Verification items for the finished model (mm, model axes). A direction names the side the tool comes from. Coordinates: 2 decimals unless noted, no trailing zeros. Order: outer loops, then holes, each group sorted by start corner. A loop starts at its lowest first (then second) coordinate and runs counter-clockwise, first axis right, second up. Notation, with made-up numbers: M 88,-20 L 139,-20 A35 cw 139,18 Z; hole C -18.5,-30 d10. An arc over 180 degrees is marked long. Answer as a JSON object with one key per item and string values. Group by question number.
(1) Material ranges on line 1 (X direction, y = 0, z = 1.65); line 2 (Y direction, x = 35, z = 2.35); line 3 (X direction, y = 0.7, z = 4.4), recorded low to high.
(2) Cross-section at A-A (x = 0). Enter the section's corners in (y, z), plus the area to 3 significant figures.
(3) Access from +Z, -Z, +X, -X, +Y, -Y to the whole of each face (thin tool, end or side, straight path). Record for faces 4 (the face through (-42.5, -0.1, 2.5)), 5 (the face through (-1, -1, 3)).
(4) Cross-section at C-C (y = 0). Count the separate pieces of the cut face and the enclosed holes in it, plus the area to 3 significant figures.
(5) Cross-section at B-B (z = 2). Enter the section's corners in (x, y).
(6) Mould release check, pull along Y, two halves, no side actions. Record for faces 1 (the face through (34, -1, 3)), 2 (the face through (0.4, 1.1, 0)), 3 (the face through (-1, 2.5, 2)): released by +Y, released by -Y, zero draft, split by the parting line, or undercut.
(7) Gauge pin test, flat ends, axial feed: pin 1 Ø1.3 at (x, y) = (35, 0.5) entering from +Z; pin 2 Ø1.1 at (x, y) = (-10, 1) entering from -Z. Record the tip position at first contact, or that the pin passes through.
from build123d import *

# Parameters (mm, degrees)
SKETCH_1_R          = 1
EXTRUDE_1_DEPTH     = 5
SKETCH_2_W          = 1
SKETCH_2_H          = 5
CUT_EXTRUDE_1_DEPTH = 0.5
SKETCH_3_R          = 2.25
CUT_EXTRUDE_3_DEPTH = 2


with BuildPart() as part:
    # 草图1 → 凸台-拉伸1 (new body)
    with BuildSketch(Plane.XY):
        with BuildLine():
            Line((-40, 2.5), (40, 2.5))
            ThreePointArc((40, 2.5), (42.500000092, 0), (40, -2.5))
            Line((40, -2.5), (-40, -2.5))
            ThreePointArc((-40, -2.5), (-42.5, 0), (-40, 2.5))
        make_face()
        with Locations((-35, 0)):
            Circle(SKETCH_1_R, mode=Mode.SUBTRACT)
        Circle(SKETCH_1_R, mode=Mode.SUBTRACT)
        with Locations((35, 0)):
            Circle(SKETCH_1_R, mode=Mode.SUBTRACT)
    extrude(amount=EXTRUDE_1_DEPTH)

    # 草图2 → 切除-拉伸1 (cut)
    with BuildSketch(Plane(origin=(0, 0, 0), x_dir=(-1, 0, 0), z_dir=(0, 0, -1))):
        with Locations((-25.5, 0)):
            Rectangle(SKETCH_2_W, SKETCH_2_H)
        with Locations((-10.5, 0)):
            Rectangle(SKETCH_2_W, SKETCH_2_H)
        with Locations((10.044565055, 0)):
            Rectangle(SKETCH_2_W, SKETCH_2_H)
        with Locations((25.5, 0)):
            Rectangle(SKETCH_2_W, SKETCH_2_H)
    extrude(amount=-CUT_EXTRUDE_1_DEPTH, mode=Mode.SUBTRACT)

    # 草图3 → 切除-拉伸3 (cut)
    with BuildSketch(Plane.XY.offset(5)):
        with Locations((-35, 0)):
            Circle(SKETCH_3_R)
        Circle(SKETCH_3_R)
        with Locations((35, 0)):
            Circle(SKETCH_3_R)
    extrude(amount=-CUT_EXTRUDE_3_DEPTH, mode=Mode.SUBTRACT)


solid = part.part
Taken from the geometry:
{
 "1": {"line 1": "x = -42.5 to -36, -34 to -1, 1 to 34, 36 to 42.5", "line 2": "y = -2.5 to -1, 1 to 2.5", "line 3": "x = -42.4 to -37.14, -32.86 to -2.14, 2.14 to 32.86, 37.14 to 42.4"},
 "2": {"outline": "M -2.5,0 L -1,0 L -1,3 L -2.25,3 L -2.25,5 L -2.5,5 Z; M 1,0 L 2.5,0 L 2.5,5 L 2.25,5 L 2.25,3 L 1,3 Z", "area": "10.0 mm²"},
 "3": {"face 4": "+Z, -Z, -X", "face 5": "+Z"},
 "4": {"separate pieces": "4", "enclosed holes": "0", "area": "378 mm²"},
 "5": {"outline": "M -40,-2.5 L 40,-2.5 A2.5 ccw 40,2.5 L -40,2.5 A2.5 ccw Z; hole C -35,0 d2; hole C 0,0 d2; hole C 35,0 d2"},
 "6": {"face 1": "undercut", "face 2": "zero draft", "face 3": "released by +Y"},
 "7": {"pin 1": "stops at z = 3", "pin 2": "stops at z = 0"}
}
